from build123d import *

# Parameters (mm, degrees)
PAD_DEPTH             = 24
POCKET_DEPTH          = 3
SKETCH002_W           = 70
SKETCH002_H           = 18.5
POCKET001_DEPTH       = 18
POLARPATTERN_COUNT    = 3
POCKET002_DEPTH       = 6
CHAMFER_SIZE          = 8
FILLET_R              = 13
FILLET001_R           = 11
CHAMFER001_SIZE       = 16.1
FILLET002_R           = 11
FILLET003_R           = 12
POCKET003_DEPTH       = 6
POCKET004_DEPTH       = 18
POCKET005_DEPTH       = 21.001
SKETCH007_W           = 15.5
SKETCH007_H           = 15
POCKET006_DEPTH       = 5
SKETCH010_W           = 13.6
SKETCH010_H           = 9
POCKET009_DEPTH       = 15.5
POCKET010_DEPTH       = 3
SKETCH012_R           = 1.85
SKETCH012_R_2         = 0.99
POCKET011_DEPTH       = 498.0492855781
POLARPATTERN001_COUNT = 3
POCKET012_DEPTH       = 12
POCKET013_DEPTH       = 3
POCKET014_DEPTH       = 3
FILLET004_R           = 2
FILLET005_R           = 1.5
FILLET006_R           = 11


with BuildPart() as part:
    # Sketch → Pad (new body)
    with BuildSketch(Plane.XY):
        Polygon((0, 112.2094915052), (-97.1762701892, -56.1047457526), (97.1762701892, -56.1047457526), align=None)
        Polygon((0, 62.2094915052), (-53.875, -31.1047457526), (53.875, -31.1047457526), align=None, mode=Mode.SUBTRACT)
    extrude(amount=PAD_DEPTH)

    # Sketch001 (on Face8 of Pad) → Pocket (cut)
    with BuildSketch(Plane.XY.offset(24)):
        Polygon((0, 98.2094915052), (-85.0519145362, -49.1047457526), (85.0519145362, -49.1047457526), align=None)
        Polygon((0, 76.2094915052), (-65.999355653, -38.1047457526), (65.999355653, -38.1047457526), align=None, mode=Mode.SUBTRACT)
    extrude(amount=-POCKET_DEPTH, mode=Mode.SUBTRACT)

    # Sketch002 (on Face4 of Pocket) → Pocket001 (cut)
    with BuildSketch(Plane(origin=(0, 0, 0), x_dir=(1, 0, 0), z_dir=(0, 0, -1))):
        with Locations((0, 43.6047457526)):
            Rectangle(SKETCH002_W, SKETCH002_H)
    pocket001 = extrude(amount=-POCKET001_DEPTH, mode=Mode.SUBTRACT)

    # PolarPattern: Pocket001 ×3 about axis
    polarpattern_axis = Axis((0, 0, 0), (0, 0, -1))
    for i in range(1, POLARPATTERN_COUNT):
        add(pocket001.rotate(polarpattern_axis, i * 360 / POLARPATTERN_COUNT), mode=Mode.SUBTRACT)

    # Sketch003 (on Face4 of PolarPattern) → Pocket002 (cut)
    with BuildSketch(Plane(origin=(0, 0, 0), x_dir=(1, 0, 0), z_dir=(0, 0, -1))):
        Polygon((0, -100.2094915052), (86.7839653438, 50.1047457526), (-86.7839653438, 50.1047457526), align=None)
        Polygon((0, -74.2094915052), (64.2673048454, 37.1047457526), (-64.2673048454, 37.1047457526), align=None, mode=Mode.SUBTRACT)
    extrude(amount=-POCKET002_DEPTH, mode=Mode.SUBTRACT)

    # Chamfer
    chamfer_edges = [part.edges().sort_by_distance(p)[0] for p in [
        (-53.875, -31.104746, 12),
        (53.875, -31.104746, 12),
        (0, 62.209492, 12),
    ]]
    chamfer(chamfer_edges, length=CHAMFER_SIZE)

    # Fillet
    fillet_edges = [part.edges().sort_by_distance(p)[0] for p in [
        (0, 100.209492, 3),
        (-86.783965, -50.104746, 3),
        (86.783965, -50.104746, 3),
    ]]
    fillet(fillet_edges, radius=FILLET_R)

    # Fillet001
    fillet001_edges = [part.edges().sort_by_distance(p)[0] for p in [
        (0, 74.209492, 3),
        (64.267305, -37.104746, 3),
        (-64.267305, -37.104746, 3),
    ]]
    fillet(fillet001_edges, radius=FILLET001_R)

    # Chamfer001
    chamfer001_edges = [part.edges().sort_by_distance(p)[0] for p in [
        (97.17627, -56.104746, 12),
        (0, 112.209492, 12),
        (-97.17627, -56.104746, 12),
    ]]
    chamfer(chamfer001_edges, length=CHAMFER001_SIZE)

    # Fillet002
    fillet002_edges = [part.edges().sort_by_distance(p)[0] for p in [
        (0, 98.209492, 22.5),
        (-85.051915, -49.104746, 22.5),
        (85.051915, -49.104746, 22.5),
    ]]
    fillet(fillet002_edges, radius=FILLET002_R)

    # Fillet003
    fillet003_edges = [part.edges().sort_by_distance(p)[0] for p in [
        (65.999356, -38.104746, 22.5),
        (0, 76.209492, 22.5),
        (-65.999356, -38.104746, 22.5),
    ]]
    fillet(fillet003_edges, radius=FILLET003_R)

    # Sketch004 (on Face60 of Fillet003) → Pocket003 (cut)
    with BuildSketch(Plane(origin=(0, 0, 6), x_dir=(1, 0, 0), z_dir=(0, 0, -1))):
        Polygon((-8.75, -72.1664825043), (8.75, -72.1664825043), (8.75, -94.7664825043), (4, -94.7664825043), (4, -98.2664825043), (-4, -98.2664825043), (-4, -94.7664825043), (-8.75, -94.7664825043), align=None)
    extrude(amount=-POCKET003_DEPTH, mode=Mode.SUBTRACT)

    # Sketch005 (on Face29 of Pocket003) → Pocket004 (cut)
    with BuildSketch(Plane(origin=(0, 0, 0), x_dir=(1, 0, 0), z_dir=(0, 0, -1))):
        Polygon((46.1715988394, 38.9547457526), (68.6882593378, 51.9547457526), (79.3382593378, 33.508404652), (56.8215988394, 20.508404652), align=None)
    extrude(amount=-POCKET004_DEPTH, mode=Mode.SUBTRACT)

    # Sketch006 (on Face1 of Pocket004) → Pocket005 (cut, through all)
    with BuildSketch(Plane.XY.offset(21)):
        with BuildLine():
            ThreePointArc((1.5, 85.0404521425), (0, 86.5404521425), (-1.5, 85.0404521425))
            Line((-1.5, 85.0404521425), (-1.5, 66.0404521425))
            ThreePointArc((-1.5, 66.0404521425), (0, 64.5404521425), (1.5, 66.0404521425))
            Line((1.5, 85.0404521425), (1.5, 66.0404521425))
        make_face()
    extrude(amount=-POCKET005_DEPTH, mode=Mode.SUBTRACT)

    # Sketch007 (on Face24 of Pocket005) → Pocket006 (cut)
    with BuildSketch(Plane(origin=(-48.5881350946, 28.0523728763, 0), x_dir=(-0.5, -0.8660254038, 0), z_dir=(-0.8660254038, 0.5, 0))):
        with Locations((-47.3262701892, 13.5)):
            Rectangle(SKETCH007_W, SKETCH007_H)
    extrude(amount=-POCKET006_DEPTH, mode=Mode.SUBTRACT)

    # Sketch010 (on Face79 of Pocket006) → Pocket009 (cut)
    with BuildSketch(Plane(origin=(-44.2580080757, 25.5523728763, 0), x_dir=(-0.5, -0.8660254038, 0), z_dir=(-0.8660254038, 0.5, 0))):
        with Locations((-47.3262701892, 13.5)):
            Rectangle(SKETCH010_W, SKETCH010_H)
    extrude(amount=-POCKET009_DEPTH, mode=Mode.SUBTRACT)

    # Sketch011 (on Face21 of Pocket009) → Pocket010 (cut)
    with BuildSketch(Plane(origin=(0, 0, 6), x_dir=(1, 0, 0), z_dir=(0, 0, -1))):
        Polygon((-21.0413798427, -59.7570681827), (-11.6817654684, -54.3532923042), (-6.658482036, -63.0538744299), (-16.0180964103, -68.4576503084), align=None)
    extrude(amount=-POCKET010_DEPTH, mode=Mode.SUBTRACT)

    # Sketch012 (on Face54 of Pocket010) → Pocket011 (cut, through all)
    with BuildSketch(Plane(origin=(0, 0, 0), x_dir=(1, 0, 0), z_dir=(0, 0, -1))):
        with Locations((-13.5, -82.7032108255)):
            Circle(SKETCH012_R)
        with Locations((13.5, -82.7032108255)):
            Circle(SKETCH012_R)
        with Locations((-6.25, -96.5164825043)):
            Circle(SKETCH012_R_2)
        with Locations((6.25, -96.5164825043)):
            Circle(SKETCH012_R_2)
        with Locations((-27.2463245869, -59.0174730012)):
            Circle(SKETCH012_R_2)
        with Locations((-47.1862074814, -27.2405827309)):
            Circle(SKETCH012_R_2)
        with Locations((-64.7337931796, 5.9127272486)):
            Circle(SKETCH012_R_2)
        with Locations((-10.791841915, -49.5174730012)):
            Circle(SKETCH012_R_2)
        with Locations((-28.3394276132, -16.3641630217)):
            Circle(SKETCH012_R_2)
        with Locations((-48.2793105078, 15.4127272487)):
            Circle(SKETCH012_R_2)
    pocket011 = extrude(amount=-POCKET011_DEPTH, mode=Mode.SUBTRACT)

    # PolarPattern001: Pocket011 ×3 about axis
    polarpattern001_axis = Axis((0, 0, 0), (0, 0, -1))
    for i in range(1, POLARPATTERN001_COUNT):
        add(pocket011.rotate(polarpattern001_axis, i * 360 / POLARPATTERN001_COUNT), mode=Mode.SUBTRACT)

    # Sketch013 (on Face132 of PolarPattern001) → Pocket012 (cut)
    with BuildSketch(Plane(origin=(0, 0, 6), x_dir=(1, 0, 0), z_dir=(0, 0, -1))):
        Polygon((58.553649647, 21.508404652), (63.3167893678, 24.258404652), (66.3167893678, 19.0622522293), (61.553649647, 16.3122522293), align=None)
    extrude(amount=-POCKET012_DEPTH, mode=Mode.SUBTRACT)

    # Sketch014 (on Face127 of Pocket012) → Pocket013 (cut)
    with BuildSketch(Plane(origin=(0, 0, 6), x_dir=(1, 0, 0), z_dir=(0, 0, -1))):
        Polygon((-74.3478338252, 33.3748379063), (-65.8478338252, 48.0972697706), (-52.8574527684, 40.5972697706), (-61.3574527684, 25.8748379063), align=None)
    extrude(amount=-POCKET013_DEPTH, mode=Mode.SUBTRACT)

    # Sketch015 (on Face21 of Pocket013) → Pocket014 (cut)
    with BuildSketch(Plane(origin=(0, 0, 6), x_dir=(1, 0, 0), z_dir=(0, 0, -1))):
        with BuildLine():
            ThreePointArc((-8.75, -63.0538744299), (-13.3063040372, -67.6101784671), (-8.75, -72.1664825043))
            Line((-8.75, -72.1664825043), (8.75, -72.1664825043))
            ThreePointArc((8.75, -72.1664825043), (13.3063040372, -67.6101784671), (8.75, -63.0538744299))
            Line((-8.75, -63.0538744299), (8.75, -63.0538744299))
        make_face()
    extrude(amount=-POCKET014_DEPTH, mode=Mode.SUBTRACT)

    # Fillet004
    fillet004_edges = [part.edges().sort_by_distance(p)[0] for p in [
        (-13.243399, 66.855678, 7.5),
    ]]
    fillet(fillet004_edges, radius=FILLET004_R)

    # Fillet005
    fillet005_edges = [part.edges().sort_by_distance(p)[0] for p in [
        (-6.658482, 63.053874, 7.5),
    ]]
    fillet(fillet005_edges, radius=FILLET005_R)

    # Fillet006
    fillet006_edges = [part.edges().sort_by_distance(p)[0] for p in [
        (-8.75, 72.166483, 7.5),
        (8.75, 72.166483, 7.5),
    ]]
    fillet(fillet006_edges, radius=FILLET006_R)


solid = part.part
Input: part model. Units: mm. Frame: model coordinates. A direction names the side the tool comes from. Coordinates: 2 decimals unless noted, no trailing zeros. Order: outer loops, then holes, each group sorted by start corner. A loop starts at its lowest first (then second) coordinate and runs counter-clockwise, first axis right, second up. Notation, with made-up numbers: M 51,81.5 L 64,81.5 A8 ccw 64,93.5 Z; hole C -37,6 d7. An arc over 180 degrees is marked long. Answer in a Markdown table with one row per item.
(1) Draft query along X for faces 4 (the flat face through (-6, 94.766, 9)), 5 (the flat face through (-1, -56.105, 12)). Return one class per face: pulls with the +X half, pulls with the -X half, needs draft (parallel to the pull), parting line crosses it, or undercut.
Numbers:
| item | result |
|---|---|
| face 4 | undercut |
| face 5 | needs draft |
(2) Material intervals for line 1 (X direction, y = 5, z = 10.5); line 2 (Y direction, x = -33, z = 17.75); line 3 (X direction, y = 39, z = 15.5), sorted ascending. Write a range as [from, to].
Numbers:
| item | result |
|---|---|
| line 1 | x = [-61.9, -58.14], [-36.78, -33.03], [33.03, 36.78], [58.14, 61.9] |
| line 2 | y = [-56.1, -52.85], [-34.35, -31.1], [5.05, 11.55], [48.55, 55.05] |
| line 3 | x = [-42.27, -38.51], [-17.15, -13.4], [13.4, 17.15], [38.51, 42.27] |
(3) Section query B-B, the plane z = 3.5. Give the number of separate pieces and of enclosed holes in the cut face, plus the area to 3 significant figures.
Numbers:
| item | result |
|---|---|
| separate pieces | 2 |
| enclosed holes | 32 |
| area | 3,930 mm^2 |
(4) Contact query for flat-ended pins moving along their axis: pin 1 Ø3 at (y, z) = (96, 10) entering from -X; pin 2 Ø4 at (y, z) = (-13, 13.5) entering from -X; pin 3 Ø1.8 at (x, y) = (47.18, 27.24) entering from +Z; pin 4 Ø1 at (x, z) = (27, 3.5) entering from +Y. Output: stop coordinate, or through.
Numbers:
| item | result |
|---|---|
| pin 1 | stops at x = -10.22 |
| pin 2 | stops at x = -73.44 |
| pin 3 | passes through |
| pin 4 | stops at y = 66.31 |
(5) Access query for faces 1 (the flat face through (-47.847, -27.689, 11.832)), 2 (the cylindrical face through (-75.61, -43.46, 22.48)), 3 (the flat face through (-55.151, -8.573, 10.874)). Directions: +Z, -Z, +X, -X, +Y, -Y. A direction counts if a zero-diameter tool reaches every point of the face in a straight line with its end or side. Return the directions, or none.
Numbers:
| item | result |
|---|---|
| face 1 | +Z, -Z |
| face 2 | +Z |
| face 3 | -Z |
(6) Section query A-A, the plane y = 11. Output: boundary loops of the cut face in (x, z).
Numbers:
| item | result |
|---|---|
| outline | M -58.43,0 L -54.68,0 L -54.68,18 L -33.32,18 L -33.32,0 L -29.57,0 L -29.57,24 L -37.65,24 L -37.65,21 L -50.35,21 L -50.35,24 L -58.43,24 Z; M 29.57,0 L 33.32,0 L 33.32,18 L 54.68,18 L 54.68,0 L 58.43,0 L 58.43,24 L 50.35,24 L 50.35,21 L 37.65,21 L 37.65,24 L 29.57,24 Z |
